```python
from build123d import *

# Parameters (mm, degrees)
F1_DEPTH       = 4
F2_D           = 4.5
F4_D           = 4.5
F4_CSINK_D     = 8.96
F4_CSINK_ANGLE = 90
F6_DEPTH       = 25


with BuildPart() as f1:
    # F0 (on Front) → F1 (new body)
    with BuildSketch(Plane.XZ):
        Polygon((16.6953813087, 0), (0, 0), (0, -80), (70, -80), (70, 0), (19.6887112585, 0), align=None)
        with BuildLine():
            ThreePointArc((12.3, -20), (13.1196675826, -18.0623854873), (15.081, -17.3012152735))
            ThreePointArc((15.081, -17.3012152735), (16.9376145127, -18.1196675826), (17.7, -20))
            ThreePointArc((17.7, -20), (23.8821053394, -42.0178946606), (40.6214035596, -57.6))
            ThreePointArc((40.6214035596, -57.6), (49.5339421791, -60.9847731931), (58.9781220381, -62.2876550004))
            ThreePointArc((58.9781220381, -62.2876550004), (60.8394880813, -63.0952428188), (61.6128496753, -64.9710875555))
            ThreePointArc((61.6128496753, -64.9710875555), (61.6128842578, -64.9789772549), (61.6128957853, -64.9868670217))
            ThreePointArc((61.6128957853, -64.9868670217), (60.7988821475, -66.9189786751), (58.8476695324, -67.686079043))
            ThreePointArc((58.8476695324, -67.686079043), (48.1978496914, -66.2168718986), (38.1475401842, -62.4))
            ThreePointArc((38.1475401842, -62.4), (19.2713102763, -44.8286897237), (12.3, -20))
        make_face(mode=Mode.SUBTRACT)
    extrude(amount=F1_DEPTH)

    # F2 (through all)
    with Locations(Plane(origin=(0, 0, 0), x_dir=(1, 0, 0), z_dir=(0, 1, 0))):
        with Locations((60, 20)):
            Hole(F2_D / 2)

    # F4 (through all)
    with Locations(Plane.XZ.offset(4)):
        with Locations((5, -5), (47, -5)):
            CounterSinkHole(F4_D / 2, F4_CSINK_D / 2, counter_sink_angle=F4_CSINK_ANGLE)

    # F5 (on face) → F6 (cut)
    with BuildSketch(Plane.XZ.offset(4)):
        Polygon((35, -80), (0, -40), (0, -80), align=None)
    extrude(amount=-F6_DEPTH, mode=Mode.SUBTRACT)


solid = f1.part
```
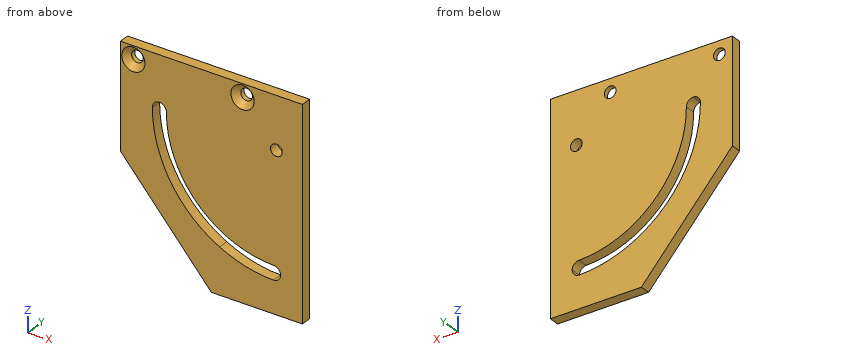
Model file for the job. Use its own axes, mm. Coordinates: 2 decimals unless noted, no trailing zeros. Loops run counter-clockwise (first coordinate to the right, second up) from the corner with the lowest first, then second, coordinate; pieces in that order, holes last. Notation, with made-up numbers: (87.25, 51.5) - (116.25, 51.5) arc R16 ccw to (116.25, 71.5) - close; hole circle Ø9 at (-26, 58). An arc over 180 degrees is marked (long way). Write item = value, one per line. Start each with the question number.
Item 1: Drop flat-ended pins along their axis: pin 1 Ø4 at (x, z) = (47, -5) entering from +Y; pin 2 Ø6 at (x, z) = (5, -5) entering from -Y. Give the stop position or say it passes through.
Item 2: Saw through at D-D, the plane z = -53. List the corners of the cut face in (x, y) (3 decimals), then the cut area to 3 significant figures.
Item 3: Saw through at A-A, the plane z = -5. List the corners of the cut face in (x, y), then the cut area to 3 significant figures.
Item 4: Wall check: probe 1 along X at (y, z) = (-0.6, -5); probe 2 along X at (y, z) = (-1.5, -20); probe 3 along Z at (x, y) = (60, -2.9). Give the ranges that are in metal, low to high. Write a range as [from, to].
Item 5: Saw through at C-C, the plane x = 56.5. List the corners of the cut face in (y, z), then the cut area to 3 significant figures.
Item 6: Saw through at B-B, the plane y = -2.7. State how many separate pieces and enclosed holes the cut face has, then the cut area to 3 significant figures.
Answers:
q1.pin_1 = through
q1.pin_2 = -2.52
q2.outline = (11.375, -4) - (25.557, -4) - (25.557, 0) - (11.375, 0) - close; (33.537, -4) - (70, -4) - (70, 0) - (33.537, 0) - close
q2.area = 203 mm2
q3.outline = (0, -4) - (0.52, -4) - (2.75, -1.77) - (2.75, 0) - (0, 0) - close; (7.25, -1.77) - (9.48, -4) - (42.52, -4) - (44.75, -1.77) - (44.75, 0) - (7.25, 0) - close; (49.25, -1.77) - (51.48, -4) - (70, -4) - (70, 0) - (49.25, 0) - close
q3.area = 234 mm2
q4.probe_1 = [0, 2.75], [7.25, 44.75], [49.25, 70]
q4.probe_2 = [0, 12.3], [17.7, 57.75], [62.25, 70]
q4.probe_3 = [-80, -67.46], [-62.52, -22.25], [-17.75, 0]
q5.outline = (-4, -80) - (0, -80) - (0, -67.57) - (-4, -67.57) - close; (-4, -62.15) - (0, -62.15) - (0, 0) - (-4, 0) - close
q5.area = 298 mm2
q6.separate_pieces = 1
q6.enclosed_holes = 4
q6.area = 4,420 mm2
